Autodesk Fusion 360 part; units mm, degrees
sketch "Sketch1" plane through (0, 0, 0) normal (0, 0, 1) x (1, 0, 0)
  line L0 (-15, -10) -> (-15, 10)
  line L1 (-15, 10) -> (15, 10)
  line L2 (15, 10) -> (15, -10)
  line L3 (15, -10) -> (-15, 10) construction
  line L4 (-15, -10) -> (15, 10) construction
  line L5 (15, -10) -> (15, -25)
  line L6 (0.0079, -14.5) -> (-15, -14.5)
  line L7 (-15, -10) -> (-15, -14.5)
  arc A0 (-10.5, -25) -> (-0.0079, -14.5) centre (0, -25) ccw
  arc A1 (-15, -25) -> (-10.7121, -14.5) centre (0, -25) ccw
  arc A2 (-10.5, -25) -> (-15, -25) centre (-12.75, -25) ccw
  line L8 (6, 6) -> (-6, 6)
  line L9 (-6, 6) -> (-6, -6)
  line L10 (-6, -6) -> (6, -6)
  line L11 (6, -6) -> (6, 6)
  line L12 (6, 6) -> (-6, -6) construction
  line L13 (-6, 6) -> (6, -6) construction
  circle A3 centre (-11.792, 0) radius 1.75
  circle A4 centre (11.792, 0) radius 1.75
  dimension "d1" = 30
  dimension "d3" = 12
  dimension "d4" = 12
  dimension "d5" = 3.5
extrude "Extrude1" add sketch "Sketch1" along normal mid plane 4 contours L0 L1 L2 L5 L6 L7 A1
extrude "Extrude2" add sketch "Sketch1" along normal mid plane 4 contours L6 A0 A1 A2
fillet "Fillet1" radius 4 2 edges at (-15, 10, 0) (15, 10, 0)
fillet "Fillet2" radius 4 1 edges at (-15, -14.5, 0)
fillet "Fillet3" radius 1 20 edges at (13.8284, 8.8284, 2) (0, 10, 2) (-13.8284, 8.8284, 2) (-15, -2.25, 2) (-13.8284, -13.3284, 2) (-5.5039, -14.5, 2) (7.4274, -32.4218, 2) (-12.75, -22.75, 2) (0, -40, 2) (15, -9.5, 2) (7.4274, -32.4218, -2) (-5.5039, -14.5, -2) (-13.8284, -13.3284, -2) (-15, -2.25, -2) (-13.8284, 8.8284, -2) (0, 10, -2) (13.8284, 8.8284, -2) (15, -9.5, -2) (0, -40, -2) (-12.75, -22.75, -2)
The model under review builds one solid part; all positions refer to its coordinate system, in mm. A direction names the side the tool comes from. Round coordinates to 2 decimals unless told otherwise and drop trailing zeros. Order: outer loops, then holes, each group sorted by start corner. A loop starts at its lowest first (then second) coordinate and runs counter-clockwise, first axis right, second up. Notation, with made-up numbers: (64, 50) -> (117, 50) arc R12 ccw to (117, 63) -> close; hole circle Ø2 at (73.25, 89). An arc over 180 degrees is marked (long way). One line per item, written item: value. Start each with the question number.
Q1. Take a section at B-B (z = -0.5). Write out the cut boundary in (x, y), and give its area (3 significant figures).
Q2. Clearance check with flat-ended pins moving along their axes: pin 1 Ø2 at (x, z) = (-5.5, 0) entering from -Y; pin 2 Ø2 at (x, y) = (4, -32.5) entering from -Z; pin 3 Ø8 at (x, y) = (-11.5, -24.5) entering from -Z; pin 4 Ø1.2 at (x, z) = (-2.5, 0.5) entering from -Y. State where each tip first meets the part, or that it passes through.
Q3. Mouldability with a two-part tool opening along Y and no side actions: class faces 4 (the face through (-5.573, -14.199, -1.715)), 5 (the face through (-14.699, -2.134, -1.715)), 6 (the face through (0.154, 9.699, -1.715)) as released by +Y, released by -Y, zero draft, split by the parting line, or undercut.
Q4. Take a section at A-A (y = 0). Write out the cut boundary in (x, z), and give its area (3 significant figures).
Q5. Wall thickness on line 1 (Y direction, x = 1.5, z = -0.45); line 2 (Y direction, x = -11, z = -0.4); line 3 (Y direction, x = 7, z = 0.3): over which ranges is each line inside the solid? List them lowest first.
Q6. Take a section at C-C (x = -1). Count the separate pieces of the cut face and the enclosed holes in it, and give its area (3 significant figures).
Q7. Machinability: for faces 1 (the face through (6, 0, 0)), 2 (the face through (14.715, -9.717, 1.699)), 3 (the face through (-5.573, -14.215, 1.699)), which of the approach directions +Z, -Z, +X, -X, +Y, -Y give a long, thin tool a straight path to every point of the face, cutting with its end or side? Answer none if there is none.
Reported:
1. outline: (-15, -25) arc R15 ccw to (15, -25) -> (15, 6) arc R4 ccw to (11, 10) -> (-11, 10) arc R4 ccw to (-15, 6) -> (-15, -10.5) arc R4 ccw to (-11, -14.5) -> (0.01, -14.5) arc R10.5 cw (long way) to (-10.5, -25) arc R2.25 ccw to start; hole circle Ø3.5 at (-11.79, 0); hole (-6, -6) -> (6, -6) -> (6, 6) -> (-6, 6) -> close; hole circle Ø3.5 at (11.79, 0)
1. area: 821 mm2
2. pin 1: stops at y = -39.31
2. pin 2: passes through
2. pin 3: stops at z = -2
2. pin 4: stops at y = -39.88
3. face 4: undercut
3. face 5: zero draft
3. face 6: released by +Y
4. outline: (-15, -1) arc R1 ccw to (-14, -2) -> (-13.54, -2) -> (-13.54, 2) -> (-14, 2) arc R1 ccw to (-15, 1) -> close; (-10.04, -2) -> (-6, -2) -> (-6, 2) -> (-10.04, 2) -> close; (6, -2) -> (10.04, -2) -> (10.04, 2) -> (6, 2) -> close; (13.54, -2) -> (14, -2) arc R1 ccw to (15, -1) -> (15, 1) arc R1 ccw to (14, 2) -> (13.54, 2) -> close
4. area: 43.1 mm2
5. line 1: y = -39.92 to -35.39, -14.61 to -6, 6 to 10
5. line 2: y = -35.2 to -23.59, -14.5 to -1.56, 1.56 to 10
5. line 3: y = -38.27 to -32.83, -17.17 to 10
6. separate pieces: 3
6. enclosed holes: 0
6. area: 66.3 mm2
7. face 1: +Z, -Z
7. face 2: +Z, +X, +Y, -Y
7. face 3: +Z, -X
